```python
from build123d import *

# Parameters (mm, degrees)
SKETCH_1_W                   = 34
SKETCH_1_H                   = 70
EXTRUDE_317_DEPTH            = 10
SKETCH_7_W                   = 15
SKETCH_7_H                   = 70
EXTRUDE_2_DEPTH              = 10
HOLE_WIZARD_M3_D             = 3.4
HOLE_WIZARD_M3_CSINK_D       = 6.3
HOLE_WIZARD_M3_CSINK_ANGLE   = 90
SKETCH_19_W                  = 32
SKETCH_19_H                  = 62
CUT_EXTRUDE_2_DEPTH          = 5
SKETCH_17_W                  = 32
SKETCH_17_H                  = 7.1
EXTRUDE_2650_DEPTH           = 0.5
SKETCH_20_W                  = 16
SKETCH_20_H                  = 70
EXTRUDE_1_DEPTH              = 10
HOLE_WIZARD_M5_2_D           = 4.2
HOLE_WIZARD_M5_2_CSINK_D     = 5.05
HOLE_WIZARD_M5_2_CSINK_ANGLE = 90
FILLET_1_R                   = 3
FILLET_3_R                   = 5
SKETCH_18_R                  = 4.3
CUT_EXTRUDE_1_DEPTH          = 0.4
FILLET_2_R                   = 2
CHAMFER_2_SIZE               = 2


with BuildPart() as part:
    # Эскиз1 → Extrude 317 (new body)
    with BuildSketch(Plane(origin=(0, 0, 0), x_dir=(1, 0, 0), z_dir=(0, 1, 0))):
        Rectangle(SKETCH_1_W, SKETCH_1_H)
    extrude(amount=-EXTRUDE_317_DEPTH)

    # Эскиз7 → База2 (add)
    with BuildSketch(Plane(origin=(0, 0, 0), x_dir=(-1, 0, 0), z_dir=(0, -1, 0))):
        with Locations((24.5, 0)):
            Rectangle(SKETCH_7_W, SKETCH_7_H)
    extrude(amount=EXTRUDE_2_DEPTH)

    # Крепление каретки M3 (through all)
    with Locations(Plane(origin=(0, 0, 0), x_dir=(-1, 0, 0), z_dir=(0, 1, 0))):
        with Locations((-12.5, -9.5), (12.5, -9.5), (12.5, 15.5), (-12.5, 15.5)):
            CounterSinkHole(HOLE_WIZARD_M3_D / 2, HOLE_WIZARD_M3_CSINK_D / 2, counter_sink_angle=HOLE_WIZARD_M3_CSINK_ANGLE)

    # Эскиз19 → Вырез-Вытянуть2 (cut)
    with BuildSketch(Plane.XZ.offset(10)):
        with Locations((0, 3)):
            Rectangle(SKETCH_19_W, SKETCH_19_H)
    extrude(amount=-CUT_EXTRUDE_2_DEPTH, mode=Mode.SUBTRACT)

    # Эскиз17 → Extrude 2650 (add)
    with BuildSketch(Plane(origin=(0, 0, 0), x_dir=(1, 0, 0), z_dir=(0, 1, 0))):
        with Locations((0, 23)):
            Rectangle(SKETCH_17_W, SKETCH_17_H)
    extrude(amount=EXTRUDE_2650_DEPTH)

    # Эскиз16 → Hole Wizard M5 (revolve, cut)
    with BuildSketch(Plane(origin=(0, -5, -23), x_dir=(0, 0, -1), z_dir=(1, 0, 0))):
        Polygon((0, 0), (0, 23.152366702), (2.75, 21.5), (2.75, 2.45), (5.2, 0), align=None)
    revolve(axis=Axis((0, -11.35, -23), (0, 1, 0)), mode=Mode.SUBTRACT)

    # Эскиз20 → Бобышка-Вытянуть1 (add)
    with BuildSketch(Plane.XZ.offset(10)):
        with Locations((-24, 0)):
            Rectangle(SKETCH_20_W, SKETCH_20_H)
    extrude(amount=EXTRUDE_1_DEPTH)

    # Hole Wizard M5 2 (through all)
    with Locations(Plane(origin=(0, 0, 0), x_dir=(-1, 0, 0), z_dir=(0, 1, 0))):
        with Locations((22, 13)):
            CounterSinkHole(HOLE_WIZARD_M5_2_D / 2, HOLE_WIZARD_M5_2_CSINK_D / 2, counter_sink_angle=HOLE_WIZARD_M5_2_CSINK_ANGLE)

    # Скругление1
    fillet_1_edges = [part.edges().sort_by_distance(p)[0] for p in [
        (17, -5, 35),
        (17, -5, -35),
    ]]
    fillet(fillet_1_edges, radius=FILLET_1_R)

    # Скругление3
    fillet_3_edges = [part.edges().sort_by_distance(p)[0] for p in [
        (-32, -10, -35),
        (-32, -10, 35),
    ]]
    fillet(fillet_3_edges, radius=FILLET_3_R)

    # Эскиз18 → Вырез-Вытянуть1 (cut)
    with BuildSketch(Plane(origin=(0, 0, 0), x_dir=(1, 0, 0), z_dir=(0, 1, 0))):
        with Locations(Location((-22, -13, 0), (0, 0, 270))):
            Circle(SKETCH_18_R)
    extrude(amount=-CUT_EXTRUDE_1_DEPTH, mode=Mode.SUBTRACT)

    # Скругление2
    fillet_2_edges = [part.edges().sort_by_distance(p)[0] for p in [
        (16, -7.5, 34),
        (16, -7.5, -28),
        (-16, -7.5, -28),
        (-16, -7.5, 34),
    ]]
    fillet(fillet_2_edges, radius=FILLET_2_R)

    # Фаска2
    # the kernel refuses this chamfer: 2 mm, written as the material it takes off along each edge
    with BuildSketch(Plane(origin=(14, 0, 32), x_dir=(0, 0, 1), z_dir=(-1, 0, 0))) as chamfer_2_piece_1:
        Polygon((3 - CHAMFER_2_SIZE, 0), (3, -CHAMFER_2_SIZE), (3, 0), align=None)
    revolve(axis=Axis((14, 0, 32), (0, 1, 0)), revolution_arc=90, mode=Mode.SUBTRACT)
    with BuildSketch(Plane(origin=(17, 0, -32), x_dir=(-0.9996219169112968, 0.027495876610586365, 0), z_dir=(0, 0, 1))) as chamfer_2_piece_2_section:
        Polygon((CHAMFER_2_SIZE * 0.999621916911, CHAMFER_2_SIZE * 0.0274958766106), (-CHAMFER_2_SIZE * 0.0274958766106, CHAMFER_2_SIZE * 0.999621916911), (0, 0), align=None)
    chamfer_2_piece_2 = extrude(amount=64, mode=Mode.PRIVATE)
    chamfer_2_piece_2 = split(chamfer_2_piece_2, bisect_by=Plane(origin=(15.636280777, -0.291141314, -26.55), z_dir=(0, 0, -1)), keep=Keep.TOP, mode=Mode.PRIVATE)
    chamfer_2_piece_2 = split(chamfer_2_piece_2, bisect_by=Plane(origin=(16, -0.291141314, -29.275), z_dir=(-1, 0, 0)), keep=Keep.TOP, mode=Mode.PRIVATE)
    add(chamfer_2_piece_2, mode=Mode.SUBTRACT)
    with BuildSketch(Plane(origin=(17, 0, -32), x_dir=(-0.9996219169112968, 0.027495876610586365, 0), z_dir=(0, 0, 1))) as chamfer_2_piece_3_section:
        Polygon((CHAMFER_2_SIZE * 0.999621916911, CHAMFER_2_SIZE * 0.0274958766106), (-CHAMFER_2_SIZE * 0.0274958766106, CHAMFER_2_SIZE * 0.999621916911), (0, 0), align=None)
    chamfer_2_piece_3 = extrude(amount=64, mode=Mode.PRIVATE)
    chamfer_2_piece_3 = split(chamfer_2_piece_3, bisect_by=Plane(origin=(16.58353142, -0.786802168, -26.55), z_dir=(0, 0, -1)), keep=Keep.TOP, mode=Mode.PRIVATE)
    chamfer_2_piece_3 = split(chamfer_2_piece_3, bisect_by=Plane(origin=(16, -0.786802168, -29.275), z_dir=(1, 0, 0)), keep=Keep.TOP, mode=Mode.PRIVATE)
    add(chamfer_2_piece_3, mode=Mode.SUBTRACT)
    with BuildSketch(Plane(origin=(17, 0, -32), x_dir=(-0.9996219169112968, 0.027495876610586365, 0), z_dir=(0, 0, 1))) as chamfer_2_piece_4_section:
        Polygon((CHAMFER_2_SIZE * 0.999621916911, CHAMFER_2_SIZE * 0.0274958766106), (-CHAMFER_2_SIZE * 0.0274958766106, CHAMFER_2_SIZE * 0.999621916911), (0, 0), align=None)
    chamfer_2_piece_4 = extrude(amount=64, mode=Mode.PRIVATE)
    chamfer_2_piece_4 = split(chamfer_2_piece_4, bisect_by=Plane(origin=(16.58353142, -0.786802168, -26.55), z_dir=(0, 0, 1)), keep=Keep.TOP, mode=Mode.PRIVATE)
    chamfer_2_piece_4 = split(chamfer_2_piece_4, bisect_by=Plane(origin=(16, -0.786802168, -23), z_dir=(1, 0, 0)), keep=Keep.TOP, mode=Mode.PRIVATE)
    chamfer_2_piece_4 = split(chamfer_2_piece_4, bisect_by=Plane(origin=(16.58353142, -0.786802168, -19.45), z_dir=(0, 0, -1)), keep=Keep.TOP, mode=Mode.PRIVATE)
    add(chamfer_2_piece_4, mode=Mode.SUBTRACT)
    with BuildSketch(Plane(origin=(17, 0, -32), x_dir=(-0.9996219169112968, 0.027495876610586365, 0), z_dir=(0, 0, 1))) as chamfer_2_piece_5_section:
        Polygon((CHAMFER_2_SIZE * 0.999621916911, CHAMFER_2_SIZE * 0.0274958766106), (-CHAMFER_2_SIZE * 0.0274958766106, CHAMFER_2_SIZE * 0.999621916911), (0, 0), align=None)
    chamfer_2_piece_5 = extrude(amount=64, mode=Mode.PRIVATE)
    chamfer_2_piece_5 = split(chamfer_2_piece_5, bisect_by=Plane(origin=(16, -0.291141314, 6.275), z_dir=(-1, 0, 0)), keep=Keep.TOP, mode=Mode.PRIVATE)
    chamfer_2_piece_5 = split(chamfer_2_piece_5, bisect_by=Plane(origin=(15.636280777, -0.291141314, -19.45), z_dir=(0, 0, 1)), keep=Keep.TOP, mode=Mode.PRIVATE)
    add(chamfer_2_piece_5, mode=Mode.SUBTRACT)
    with BuildSketch(Plane(origin=(17, 0, -32), x_dir=(-0.9996219169112968, 0.027495876610586365, 0), z_dir=(0, 0, 1))) as chamfer_2_piece_6_section:
        Polygon((CHAMFER_2_SIZE * 0.999621916911, CHAMFER_2_SIZE * 0.0274958766106), (-CHAMFER_2_SIZE * 0.0274958766106, CHAMFER_2_SIZE * 0.999621916911), (0, 0), align=None)
    chamfer_2_piece_6 = extrude(amount=64, mode=Mode.PRIVATE)
    chamfer_2_piece_6 = split(chamfer_2_piece_6, bisect_by=Plane(origin=(16, -0.786802168, 6.275), z_dir=(1, 0, 0)), keep=Keep.TOP, mode=Mode.PRIVATE)
    chamfer_2_piece_6 = split(chamfer_2_piece_6, bisect_by=Plane(origin=(16.58353142, -0.786802168, -19.45), z_dir=(0, 0, 1)), keep=Keep.TOP, mode=Mode.PRIVATE)
    add(chamfer_2_piece_6, mode=Mode.SUBTRACT)
    with BuildSketch(Plane(origin=(14, 0, -32), x_dir=(0, 0, -1), z_dir=(-1, 0, 0))) as chamfer_2_piece_7:
        Polygon((3 - CHAMFER_2_SIZE, 0), (3, CHAMFER_2_SIZE), (3, 0), align=None)
    revolve(axis=Axis((14, 0, -32), (0, -1, 0)), revolution_arc=90, mode=Mode.SUBTRACT)
    with BuildSketch(Plane(origin=(-27, 0, -35), x_dir=(0, 0.02749587661058639, 0.9996219169112968), z_dir=(1, 0, 0))) as chamfer_2_piece_8:
        Polygon((CHAMFER_2_SIZE * 0.999621916911, CHAMFER_2_SIZE * 0.0274958766106), (-CHAMFER_2_SIZE * 0.0274958766106, CHAMFER_2_SIZE * 0.999621916911), (0, 0), align=None)
    extrude(amount=41, mode=Mode.SUBTRACT)
    with BuildSketch(Plane(origin=(-32, 0, -30), x_dir=(0.9996219169112968, 0.02749587661058639, 0), z_dir=(0, 0, 1))) as chamfer_2_piece_9:
        Polygon((CHAMFER_2_SIZE * 0.999621916911, -CHAMFER_2_SIZE * 0.0274958766106), (-CHAMFER_2_SIZE * 0.0274958766106, -CHAMFER_2_SIZE * 0.999621916911), (0, 0), align=None)
    extrude(amount=60, mode=Mode.SUBTRACT)
    with BuildSketch(Plane(origin=(-27, 0, 35), x_dir=(0, 0.027495876610586296, -0.9996219169112968), z_dir=(1, 0, 0))) as chamfer_2_piece_10:
        Polygon((CHAMFER_2_SIZE * 0.999621916911, -CHAMFER_2_SIZE * 0.0274958766106), (-CHAMFER_2_SIZE * 0.0274958766106, -CHAMFER_2_SIZE * 0.999621916911), (0, 0), align=None)
    extrude(amount=41, mode=Mode.SUBTRACT)
    with BuildSketch(Plane(origin=(-27, 0, -30), x_dir=(0, 0, -1), z_dir=(1, 0, 0))) as chamfer_2_piece_11:
        Polygon((5 - CHAMFER_2_SIZE, 0), (5, -CHAMFER_2_SIZE), (5, 0), align=None)
    revolve(axis=Axis((-27, 0, -30), (0, 1, 0)), revolution_arc=90, mode=Mode.SUBTRACT)
    with BuildSketch(Plane(origin=(-27, 0, 30), x_dir=(-1, 0, 0), z_dir=(0, 0, -1))) as chamfer_2_piece_12:
        Polygon((5 - CHAMFER_2_SIZE, 0), (5, -CHAMFER_2_SIZE), (5, 0), align=None)
    revolve(axis=Axis((-27, 0, 30), (0, 1, 0)), revolution_arc=90, mode=Mode.SUBTRACT)


solid = part.part
```
For this review, take the finished solid that the model builds, in its own axes (mm). A direction names the side the tool comes from. Coordinates: 2 decimals unless noted, no trailing zeros. Loops run counter-clockwise (first coordinate to the right, second up) from the corner with the lowest first, then second, coordinate; pieces in that order, holes last.
1. Add section D-D, the plane x = -12.5. Give the boundary of the cut face in (y, z).
2. Mouldability with a two-part tool opening along X and no side actions: class faces 5 (the cylindrical face through (-11.7, -3.2, -11)), 6 (the flat face through (-31, -1, 0)), 7 (the flat face through (-7, -1, 34)), 8 (the flat face through (16, -1, 0)) as +X half, -X half, draft (parallel to the pull), parting line (faces both ways), or undercut.
3. For faces 1 (the flat face through (4, -10, -29)), 2 (the conical face through (-29.71, -0.79, 32.65)), 3 (the flat face through (16, 0, -23)), 4 (the flat face through (0, -5, 3)), list the 3-axis set-ups (+Z, -Z, +X, -X, +Y, -Y) from which the entire face can be reached by the end or side of a thin tool; tool diameter is ignored.
4. Add section B-B, the plane z = -23. Give the boundary of the cut face in (x, y).
5. For line 1 (Z direction, x = -12.5, y = -2.2); line 2 (X direction, y = -2.75, z = -9.5); line 3 (X direction, y = -16, z = 13), list the stretches that pass through material, from the lowest coordinate up.
6. Add section C-C, the plane y = -12.5. Give the boundary of the cut face in (x, z).
7. Insertion check: P1, Ø10, axis at x = 5, z = -3, coming from the -Y side; P2, Ø1.5, axis at x = -8.5, z = -9.5, coming from the +Y side; P3, Ø4.5, axis at x = 12.5, z = 15.5, coming from the +Y side; P4, Ø2, axis at x = -12.5, z = 15.5, coming from the -Y side. Each pin has a flat end and moves straight along its axis. Give the tip position at first contact, or say it passes through.
8. Add section A-A, the plane x = 0. Give the boundary of the cut face in (y, z).
Result:
1. outline: (-10, -35) - (-2, -35) - (0, -33) - (0, -26.55) - (0.5, -26.55) - (0.5, -19.45) - (0, -19.45) - (0, -12.65) - (-1.45, -11.2) - (-5, -11.2) - (-5, -28) - (-10, -28) - close; (-10, 34) - (-5, 34) - (-5, 17.2) - (-1.45, 17.2) - (0, 18.65) - (0, 33) - (-2, 35) - (-10, 35) - close; (-5, -7.8) - (-1.45, -7.8) - (0, -6.35) - (0, 12.35) - (-1.45, 13.8) - (-5, 13.8) - close
2. face 5: undercut
2. face 6: -X half
2. face 7: draft
2. face 8: +X half
3. face 1: +Z, -Z, +X, -Y
3. face 2: +Z, -X, +Y
3. face 3: +Z, -Z, +X, +Y
3. face 4: -Y
4. outline: (-32, -20) - (-16, -20) - (-16, -5) - (-5.2, -5) - (-2.75, -2.55) - (-2.75, 0.5) - (-16, 0.5) - (-16, 0) - (-30, 0) - (-32, -2) - close; (2.75, -2.55) - (5.2, -5) - (16, -5) - (16, -10) - (17, -10) - (17, -2) - (16, -1) - (16, 0.5) - (2.75, 0.5) - close
5. line 1: z = -35 to -11.2, -7.8 to 13.8, 17.2 to 35
5. line 2: x = -32 to -14.2, -10.8 to 10.8, 14.2 to 17
5. line 3: x = -32 to -24.1, -19.9 to -16
6. outline: (-32, -30) arc R5 ccw to (-27, -35) - (-16, -35) - (-16, 35) - (-27, 35) arc R5 ccw to (-32, 30) - close; hole circle Ø4.2 at (-22, 13)
7. P1: stops at y = -5
7. P2: stops at y = 0
7. P3: stops at y = -0.9
7. P4: passes through
8. outline: (-10, -35) - (-2, -35) - (0, -33) - (0, -26.55) - (0.5, -26.55) - (0.5, -25.75) - (-2.55, -25.75) - (-5, -28.2) - (-5, -28) - (-10, -28) - close; (-10, 34) - (-5, 34) - (-5, -17.8) - (-2.55, -20.25) - (0.5, -20.25) - (0.5, -19.45) - (0, -19.45) - (0, 33) - (-2, 35) - (-10, 35) - close
